from build123d import *

# Parameters (mm, degrees)
SKETCH1_W           = 127
SKETCH1_H           = 177.8
BOSS_EXTRUDE1_DEPTH = 3.175
SKETCH7_W           = 127
SKETCH7_H           = 69.425000088
CUT_EXTRUDE5_DEPTH  = 110.295656936
SKETCH8_W           = 3.175
SKETCH8_H           = 108.374999912
BOSS_EXTRUDE2_DEPTH = 3.175
SKETCH9_W           = 46.99
SKETCH9_H           = 74.422
CUT_EXTRUDE6_DEPTH  = 112.17034789
FILLET1_R           = 1.5875
SKETCH10_R          = 3.175
CUT_EXTRUDE7_DEPTH  = 112.17034789


with BuildPart() as part:
    # Sketch1 → Boss-Extrude1 (new body)
    with BuildSketch(Plane(origin=(0, 0, 0), x_dir=(0, 0, -1), z_dir=(1, 0, 0))):
        Rectangle(SKETCH1_W, SKETCH1_H)
    extrude(amount=-BOSS_EXTRUDE1_DEPTH)

    # Sketch7 → Cut-Extrude5 (cut, through all)
    with BuildSketch(Plane(origin=(0, 0, 0), x_dir=(0, 0, -1), z_dir=(1, 0, 0))):
        with Locations((0, 54.187499956)):
            Rectangle(SKETCH7_W, SKETCH7_H)
    extrude(amount=-CUT_EXTRUDE5_DEPTH, mode=Mode.SUBTRACT)

    # Sketch8 → Boss-Extrude2 (add)
    with BuildSketch(Plane(origin=(0, 0, 0), x_dir=(0, 0, -1), z_dir=(1, 0, 0))):
        with Locations((-65.0875, -34.712500044)):
            Rectangle(SKETCH8_W, SKETCH8_H)
        with Locations((65.0875, -34.712500044)):
            Rectangle(SKETCH8_W, SKETCH8_H)
    extrude(amount=-BOSS_EXTRUDE2_DEPTH)

    # Sketch9 → Cut-Extrude6 (cut, through all)
    with BuildSketch(Plane(origin=(0, 0, 0), x_dir=(0, 0, -1), z_dir=(1, 0, 0))):
        with Locations((0, -47.879)):
            Rectangle(SKETCH9_W, SKETCH9_H)
    extrude(amount=-CUT_EXTRUDE6_DEPTH, mode=Mode.SUBTRACT)

    # Fillet1
    fillet1_edges = [part.edges().sort_by_distance(p)[0] for p in [
        (0, -10.668, 0),
        (0, -85.09, 0),
        (0, -47.879, 23.495),
        (0, -47.879, -23.495),
    ]]
    fillet(fillet1_edges, radius=FILLET1_R)

    # Sketch10 → Cut-Extrude7 (cut, through all)
    with BuildSketch(Plane(origin=(0, 0, 0), x_dir=(0, 0, -1), z_dir=(1, 0, 0))):
        with Locations((-57.15, -60.325)):
            Circle(SKETCH10_R)
        with Locations((-57.15, -12.275000088)):
            Circle(SKETCH10_R)
        with Locations((-34.925, 9.949999912)):
            Circle(SKETCH10_R)
        with Locations(Location((34.925, 9.949999912, 0), (0, 0, 180))):
            Circle(SKETCH10_R)
        with Locations(Location((57.15, -12.275000088, 0), (0, 0, 180))):
            Circle(SKETCH10_R)
        with Locations(Location((57.15, -60.325, 0), (0, 0, 180))):
            Circle(SKETCH10_R)
    extrude(amount=-CUT_EXTRUDE7_DEPTH, mode=Mode.SUBTRACT)


solid = part.part
Can you work these out from the model? Positions are in its coordinate system, mm. Round coordinates to 2 decimals unless told otherwise and drop trailing zeros. Write each loop counter-clockwise with the first axis right and the second up, starting at its lowest first coordinate (ties: lowest second). Pieces come first, ordered by that corner, then holes. Notation, with made-up numbers: (63, 32) -> (75, 32) arc R18 ccw to (75, 58) -> close; hole circle Ø4 at (44.5, 27). An arc over 180 degrees is marked (long way). Use one line per item in the form item = value. Start each with the question number.
Q1. Imagine slicing it at A-A (z = 21). Please give me the cut outline in (x, y) (1 decimal), then the cut area to 3 significant figures.
Q2. Imagine slicing it at D-D (x = -2.15). Please give me the cut outline in (y, z) (3 decimals).
Q3. We'd pull the mould along Y, two halves only. Please class faces 1 (the face through (-2, 19.475, 1)), 2 (the face through (-2, -35, 66.675)), 3 (the face through (-1.565, 10.904, 31.897)), 4 (the face through (-2, -88.9, 1)): +Y half, -Y half, draft (parallel to the pull), parting line (faces both ways), or undercut.
Q4. Imagine slicing it at C-C (z = -57.15). Please give me the cut outline in (x, y) (3 decimals), then the cut area to 3 significant figures.
Q5. If I drill on probe 1 along Y at (x, z) = (-1.65, 57.15) (3 decimals); probe 2 along Z at (x, y) = (-2.05, -40) (3 decimals); probe 3 along Z at (x, y) = (-1.7, -62) (3 decimals), over which ranges is the centre line in solid material (lowest first)? Write a range as [from, to].
Q6. Imagine slicing it at B-B (y = -21). Please give me the cut outline in (x, z) (1 decimal), then the cut area to 3 significant figures.
Worked out:
q1.outline = (-3.2, -88.9) -> (0, -88.9) -> (0, -86.7) arc R1.6 ccw to (-1.6, -85.1) -> (-3.2, -85.1) -> close; (-3.2, -10.7) -> (-1.6, -10.7) arc R1.6 ccw to (0, -9.1) -> (0, 19.5) -> (-3.2, 19.5) -> close
q1.area = 107 mm^2
q2.outline = (-88.9, -66.675) -> (19.475, -66.675) -> (19.475, 66.675) -> (-88.9, 66.675) -> close; hole (-85.09, -23.495) -> (-10.668, -23.495) -> (-10.668, 23.495) -> (-85.09, 23.495) -> close; hole circle Ø6.35 at (-60.325, -57.15); hole circle Ø6.35 at (-60.325, 57.15); hole circle Ø6.35 at (-12.275, -57.15); hole circle Ø6.35 at (-12.275, 57.15); hole circle Ø6.35 at (9.95, -34.925); hole circle Ø6.35 at (9.95, 34.925)
q3.face_1 = +Y half
q3.face_2 = draft
q3.face_3 = undercut
q3.face_4 = -Y half
q4.outline = (-3.175, -88.9) -> (0, -88.9) -> (0, -63.5) -> (-3.175, -63.5) -> close; (-3.175, -57.15) -> (0, -57.15) -> (0, -15.45) -> (-3.175, -15.45) -> close; (-3.175, -9.1) -> (0, -9.1) -> (0, 19.475) -> (-3.175, 19.475) -> close
q4.area = 304 mm^2
q5.probe_1 = [-88.9, -63.5], [-57.15, -15.45], [-9.1, 19.475]
q5.probe_2 = [-66.675, -23.495], [23.495, 66.675]
q5.probe_3 = [-66.675, -59.847], [-54.453, -23.495], [23.495, 54.453], [59.847, 66.675]
q6.outline = (-3.2, -66.7) -> (0, -66.7) -> (0, -25.1) arc R1.6 ccw to (-1.6, -23.5) -> (-3.2, -23.5) -> close; (-3.2, 23.5) -> (-1.6, 23.5) arc R1.6 ccw to (0, 25.1) -> (0, 66.7) -> (-3.2, 66.7) -> close
q6.area = 273 mm^2
